Autodesk Inventor part; units mm, degrees
ref_plane "YZ Plane" through (0, 0, 0) normal (1, 0, 0) x (0, 1, 0)
ref_plane "XZ Plane" through (0, 0, 0) normal (0, 1, 0) x (-1, 0, 0)
ref_plane "XY Plane" through (0, 0, 0) normal (0, 0, 1) x (1, 0, 0)
sketch "スケッチ1" plane through (0, 0, 0) normal (1, 0, 0) x (0, 1, 0)
  line L0 (10.9, 20) -> (10.9, 0)
  line L1 (10.9, 0) -> (10, 0)
  line L2 (10, 0) -> (10, -20)
  line L3 (10, -20) -> (20.9, -20)
  line L4 (0, -28) -> (0, 28)
  line L5 (10.9, 20) -> (20.9, 20)
  line L6 (20.9, 20) -> (20.9, -20)
  point P0 (0, 0)
  dimension "d1" = 10
  dimension "d2" = 20
  dimension "d3" = 10.9
  dimension "d14" = 20.9
  dimension "d15" = 20
revolve "回転1" add sketch "スケッチ1" angle 360 about axis through (0, 0, -10) along (0, 0, 1)
thread "ねじ1"
chamfer "面取り1" distance 33 distance2 9 1 edges at (0, -20.9, 20) measured on face at (1.6818, 20.8322, -6.6667)
chamfer "面取り2" distance 4 angle 45 1 edges at (0, -20.9, -20)
properties part number "rod390_end_cap" material "ステンレス鋼"
Design review of the part built by this model. Coordinates are the model's own, in mm. A direction names the side the tool comes from. Give positions to 0.01 mm unless a question says otherwise; leave off trailing zeros. Order: outer loops, then holes, each group sorted by start corner. A loop starts at its lowest first (then second) coordinate and runs counter-clockwise, first axis right, second up. Notation, with made-up numbers: M 74,9.25 L 120,9.25 A12 ccw 120,30.25 Z; hole C 21,60 d5. An arc over 180 degrees is marked long. One line per question, with ' | ' between items. Start each with the question number.
Q1. For L1, parallel to X at y = 0, z = -13.5; L2, parallel to X at y = 0, z = 6.5; L3, parallel to Y at x = 0, z = -12.25, list the stretches that pass through material, from the lowest coordinate up. Write a range as [from, to].
Q2. We need section C-C (z = -14). Write out the cut boundary in (x, y), plus the area to 3 significant figures.
Q3. Machinability: for faces 1 (the face through (16.74, -3.72, -19.75)), 2 (the face through (3.27, 10.4, 9.86)), which of the approach directions +Z, -Z, +X, -X, +Y, -Y give a long, thin tool a straight path to every point of the face, cutting with its end or side? Answer none if there is none.
Q4. For pin 1 Ø1 at (y, z) = (10, 12) entering from +X; pin 2 Ø17.5 at (x, y) = (-5, 2.5) entering from +Z; pin 3 Ø6 at (y, z) = (-5, 9.5) entering from +X; pin 4 Ø3 at (x, z) = (-16.5, -15.5) entering from +Y, all flat-tipped, find the tip position at first contact; note any pin that passes through.
Q5. The part is to be moulded in two halves that separate along X. For faces 3 (the face through (10, 5, 20)), 4 (the face through (14.13, -15.4, -14.52)), 5 (the face through (9, 5, 0)), 6 (the face through (-9.76, -2.17, -10.14)), say which applies: +X half, -X half, draft (parallel to the pull), parting line (faces both ways), or undercut.
Q6. We need section A-A (x = 0). Write out the cut boundary in (y, z), plus the area to 3 significant figures.
Q7. We need section D-D (z = 5.5). Write out the cut boundary in (x, y), plus the area to 3 significant figures.
Returned:
1) L1: [-20.9, -10], [10, 20.9] | L2: [-15.58, -10.9], [10.9, 15.58] | L3: [-20.7, -10], [10, 20.7]
2) outline: C 0,0 d41.8; hole C 0,0 d20 | area: 1,060 mm2
3) face 1: -Z | face 2: +Z
4) pin 1: x = 10.43 | pin 2: z = 20 | pin 3: x = 15.08 | pin 4: y = 14.55
5) face 3: draft | face 4: parting line | face 5: undercut | face 6: undercut
6) outline: M -20.9,-16 L -16.9,-20 L -10,-20 L -10,0 L -10.9,0 L -10.9,20 L -11.9,20 L -20.9,-13 Z; M 10,-20 L 16.9,-20 L 20.9,-16 L 20.9,-13 L 11.9,20 L 10.9,20 L 10.9,0 L 10,0 Z | area: 523 mm2
7) outline: C 0,0 d31.71; hole C 0,0 d21.8 | area: 416 mm2
